Part model, mm, in its own coordinate system. Face numbers are marked on the shaded views. Give positions to 0.01 mm unless a question says otherwise; leave off trailing zeros. Write each loop counter-clockwise with the first axis right and the second up, starting at its lowest first coordinate (ties: lowest second). Pieces come first, ordered by that corner, then holes. Notation, with made-up numbers: M 29,63 L 67,63 A19 ccw 67,88 Z; hole C 55,-28.75 d10. An arc over 180 degrees is marked long. Use a Markdown table: item, result.
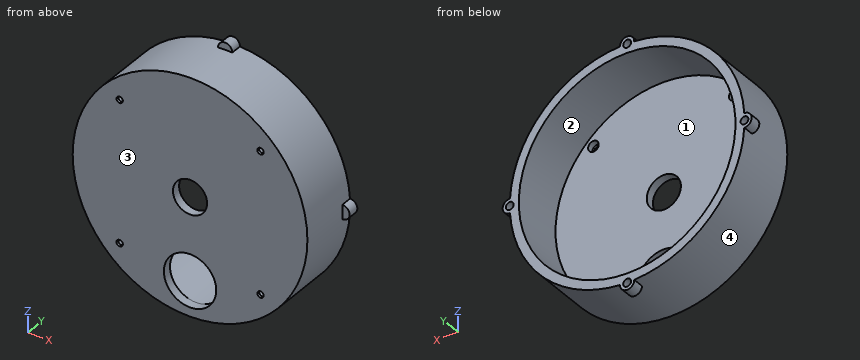
```python
from build123d import *

# Parameters (mm, degrees)
SKETCH1_R           = 82.55
SKETCH1_R_2         = 18.415
SKETCH1_R_3         = 12
BOSS_EXTRUDE1_DEPTH = 6.35
BOSS_EXTRUDE2_START = 38.1
SKETCH1_3_R         = 82.55
SKETCH1_3_R_2       = 76.2
BOSS_EXTRUDE2_DEPTH = 38.1
SKETCH5_R           = 3.75
SKETCH5_R_2         = 2.25
CUT_EXTRUDE1_DEPTH  = 4.5
SKETCH5_4_R         = 2.25
CUT_EXTRUDE2_DEPTH  = 12.7
SKETCH6_R           = 5
BOSS_EXTRUDE3_DEPTH = 8
SKETCH6_3_R         = 2.75
CUT_EXTRUDE3_DEPTH  = 7


with BuildPart() as part:
    # Sketch1 → Boss-Extrude1 (new body)
    with BuildSketch(Plane(origin=(0, 0, 0), x_dir=(1, 0, 0), z_dir=(0, 1, 0))):
        with Locations(Location((0, 0, 0), (0, 0, 270))):
            Circle(SKETCH1_R)
        with Locations(Location((0, 57.785, 0), (0, 0, 270))):
            Circle(SKETCH1_R_2, mode=Mode.SUBTRACT)
        with Locations(Location((0, 0, 0), (0, 0, 270))):
            Circle(SKETCH1_R_3, mode=Mode.SUBTRACT)
    extrude(amount=-BOSS_EXTRUDE1_DEPTH)

    # Sketch1_3 → Boss-Extrude2 (add)
    with BuildSketch(Plane(origin=(0, 0, 0), x_dir=(1, 0, 0), z_dir=(0, 1, 0)).offset(BOSS_EXTRUDE2_START)):
        with Locations(Location((0, 0, 0), (0, 0, 270))):
            Circle(SKETCH1_3_R)
        with Locations(Location((0, 0, 0), (0, 0, 89.999947602))):
            Circle(SKETCH1_3_R_2, mode=Mode.SUBTRACT)
    extrude(amount=-BOSS_EXTRUDE2_DEPTH)

    # Sketch5 → Cut-Extrude1 (cut)
    # profile 1 of 4: a face of its own
    with BuildSketch(Plane(origin=(0, 0, 0), x_dir=(1, 0, 0), z_dir=(0, 1, 0))):
        with Locations(Location((-49.53, 49.53, 0), (0, 0, 270))):
            Circle(SKETCH5_R)
        with Locations(Location((-49.53, 49.53, 0), (0, 0, 270))):
            Circle(SKETCH5_R_2, mode=Mode.SUBTRACT)
    # profile 2 of 4: a face of its own
    with BuildSketch(Plane(origin=(0, 0, 0), x_dir=(1, 0, 0), z_dir=(0, 1, 0))):
        with Locations(Location((49.53, 49.53, 0), (0, 0, 270))):
            Circle(SKETCH5_R)
        with Locations(Location((49.53, 49.53, 0), (0, 0, 270))):
            Circle(SKETCH5_R_2, mode=Mode.SUBTRACT)
    # profile 3 of 4: a face of its own
    with BuildSketch(Plane(origin=(0, 0, 0), x_dir=(1, 0, 0), z_dir=(0, 1, 0))):
        with Locations(Location((49.53, -49.53, 0), (0, 0, 270))):
            Circle(SKETCH5_R)
        with Locations(Location((49.53, -49.53, 0), (0, 0, 270))):
            Circle(SKETCH5_R_2, mode=Mode.SUBTRACT)
    # profile 4 of 4: a face of its own
    with BuildSketch(Plane(origin=(0, 0, 0), x_dir=(1, 0, 0), z_dir=(0, 1, 0))):
        with Locations(Location((-49.53, -49.53, 0), (0, 0, 270))):
            Circle(SKETCH5_R)
        with Locations(Location((-49.53, -49.53, 0), (0, 0, 270))):
            Circle(SKETCH5_R_2, mode=Mode.SUBTRACT)
    extrude(amount=-CUT_EXTRUDE1_DEPTH, mode=Mode.SUBTRACT)

    # Sketch5_4 → Cut-Extrude2 (cut)
    with BuildSketch(Plane(origin=(0, 0, 0), x_dir=(1, 0, 0), z_dir=(0, 1, 0))):
        with Locations(Location((-49.53, -49.53, 0), (0, 0, 270))):
            Circle(SKETCH5_4_R)
        with Locations(Location((49.53, -49.53, 0), (0, 0, 270))):
            Circle(SKETCH5_4_R)
        with Locations(Location((49.53, 49.53, 0), (0, 0, 270))):
            Circle(SKETCH5_4_R)
        with Locations(Location((-49.53, 49.53, 0), (0, 0, 270))):
            Circle(SKETCH5_4_R)
    extrude(amount=-CUT_EXTRUDE2_DEPTH, mode=Mode.SUBTRACT)

    # Sketch6 → Boss-Extrude3 (add)
    with BuildSketch(Plane(origin=(0, 38.1, 0), x_dir=(1, 0, 0), z_dir=(0, 1, 0))):
        with Locations((-82.55, 0)):
            Circle(SKETCH6_R)
        with Locations((0, 82.55)):
            Circle(SKETCH6_R)
        with Locations((82.55, 0)):
            Circle(SKETCH6_R)
        with Locations((0, -82.55)):
            Circle(SKETCH6_R)
    extrude(amount=-BOSS_EXTRUDE3_DEPTH)

    # Sketch6_3 → Cut-Extrude3 (cut)
    with BuildSketch(Plane(origin=(0, 38.1, 0), x_dir=(1, 0, 0), z_dir=(0, 1, 0))):
        with Locations(Location((-82.55, 0, 0), (0, 0, 270))):
            Circle(SKETCH6_3_R)
        with Locations(Location((0, 82.55, 0), (0, 0, 270))):
            Circle(SKETCH6_3_R)
        with Locations(Location((82.55, 0, 0), (0, 0, 270))):
            Circle(SKETCH6_3_R)
        with Locations(Location((0, -82.55, 0), (0, 0, 270))):
            Circle(SKETCH6_3_R)
    extrude(amount=-CUT_EXTRUDE3_DEPTH, mode=Mode.SUBTRACT)


solid = part.part
```
1. Cut at A-A, the plane z = 0. Give the cut face in (x, y).
Findings below:
| item | result |
|---|---|
| outline | M -87.55,30.1 L -82.55,30.1 L -82.55,-6.35 L -12,-6.35 L -12,0 L -76.2,0 L -76.2,38.1 L -79.8,38.1 L -79.8,31.1 L -85.3,31.1 L -85.3,38.1 L -87.55,38.1 Z; M 12,-6.35 L 82.55,-6.35 L 82.55,30.1 L 87.55,30.1 L 87.55,38.1 L 85.3,38.1 L 85.3,31.1 L 79.8,31.1 L 79.8,38.1 L 76.2,38.1 L 76.2,0 L 12,0 Z |
2. Cut at C-C, the plane x = -21. Give the cut face in (y, z), then the cut area to 3 significant figures.
Findings below:
| item | result |
|---|---|
| outline | M -6.35,-79.83 L 38.1,-79.83 L 38.1,-73.25 L 0,-73.25 L 0,73.25 L 38.1,73.25 L 38.1,79.83 L -6.35,79.83 Z |
| area | 1,520 mm2 |
3. Drop flat-ended pins along their axis: P1, Ø8, axis at x = 50.5, z = -48, coming from the +Y side; P2, Ø6, axis at x = -24.5, y = 10.5, coming from the +Z side; P3, Ø8.5, axis at x = 49.53, z = -49.53, coming from the -Y side; P4, Ø2.5, axis at x = -0.5, z = -85.5, coming from the -Y side. Give the stop position or say it passes through.
Findings below:
| item | result |
|---|---|
| P1 | y = 0 |
| P2 | z = 79.7 |
| P3 | y = -6.35 |
| P4 | y = 30.1 |
4. Two-plate mould, pull along X, no slides. Class the marked faces 1, 2, 3 and 4: released by +X, released by -X, zero draft, split by the parting line, or undercut.
Findings below:
| item | result |
|---|---|
| face 1 | undercut |
| face 2 | undercut |
| face 3 | zero draft |
| face 4 | split by the parting line |
5. Cut at B-B, the plane z = -49.53. Give the cut face in (x, y).
Findings below:
| item | result |
|---|---|
| outline | M -66.04,-6.35 L -51.78,-6.35 L -51.78,-4.5 L -53.28,-4.5 L -53.28,0 L -57.91,0 L -57.91,38.1 L -66.04,38.1 Z; M -47.28,-6.35 L -16.46,-6.35 L -16.46,0 L -45.78,0 L -45.78,-4.5 L -47.28,-4.5 Z; M 16.46,-6.35 L 47.28,-6.35 L 47.28,-4.5 L 45.78,-4.5 L 45.78,0 L 16.46,0 Z; M 51.78,-6.35 L 66.04,-6.35 L 66.04,38.1 L 57.91,38.1 L 57.91,0 L 53.28,0 L 53.28,-4.5 L 51.78,-4.5 Z |
6. Cut at D-D, the plane z = 49.53. Give the cut face in (x, y).
Findings below:
| item | result |
|---|---|
| outline | M -66.04,-6.35 L -51.78,-6.35 L -51.78,-4.5 L -53.28,-4.5 L -53.28,0 L -57.91,0 L -57.91,38.1 L -66.04,38.1 Z; M -47.28,-6.35 L 47.28,-6.35 L 47.28,-4.5 L 45.78,-4.5 L 45.78,0 L -45.78,0 L -45.78,-4.5 L -47.28,-4.5 Z; M 51.78,-6.35 L 66.04,-6.35 L 66.04,38.1 L 57.91,38.1 L 57.91,0 L 53.28,0 L 53.28,-4.5 L 51.78,-4.5 Z |
7. Drill centre lines: L1, parallel to X at y = 33.25, z = 0; L2, parallel to X at y = -3, z = 49; L3, parallel to X at y = 23, z = 0. Where is each one in solid material? Low to high.
Findings below:
| item | result |
|---|---|
| L1 | -87.55 to -85.3, -79.8 to -76.2, 76.2 to 79.8, 85.3 to 87.55 |
| L2 | -66.43 to -53.24, -45.82 to 45.82, 53.24 to 66.43 |
| L3 | -82.55 to -76.2, 76.2 to 82.55 |
